Autodesk Inventor part; units mm, degrees
ref_plane "YZ Plane" through (0, 0, 0) normal (1, 0, 0) x (0, 1, 0)
ref_plane "XZ Plane" through (0, 0, 0) normal (0, 1, 0) x (-1, 0, 0)
ref_plane "XY Plane" through (0, 0, 0) normal (0, 0, 1) x (1, 0, 0)
ref_plane "Work Plane1" through (469.0633, -361.0645, -298.4444) normal (0, 1, 0) x (0, 0, 1)
sketch "Sketch2" plane through (469.0633, -361.0645, -298.4444) normal (0, 1, 0) x (0, 0, 1)
  circle A0 centre (0, 0) radius 3
  point P0 (298.4444, -469.0633)
  dimension "d6" = 6
extrude "Extrusion1" add sketch "Sketch2" along normal blind 251
sketch "Sketch5" plane through (469.0633, -110.0645, -298.4444) normal (0, 1, 0) x (1, 0, 0)
  circle A0 centre (0, 0) radius 3
  circle A1 centre (0, 0) radius 1.5
  point P0 (-469.0633, -298.4444)
  dimension "d26" = 3
extrude "Extrusion2" add sketch "Sketch5" along normal blind 4.7 contours A1
sketch "Sketch6" plane through (469.0633, -105.3645, -298.4444) normal (0, 1, 0) x (1, 0, 0)
  circle A0 centre (0, 0) radius 1.5
  circle A1 centre (0, 0) radius 2
  point P0 (-469.0633, -298.4444)
  dimension "d29" = 4
extrude "Extrusion3" add sketch "Sketch6" against normal blind 3.7
thread "Thread1"
chamfer "Chamfer2" distance 0.3 angle 45 1 edges at (467.0633, -105.3645, -298.4444)
sketch "Sketch7" plane through (469.0633, -361.0645, -298.4444) normal (0, -1, 0) x (1, 0, 0)
  circle A0 centre (0, 0) radius 3
  circle A1 centre (0, 0) radius 1.5
  point P0 (-469.0633, 298.4444)
  dimension "d37" = 3
extrude "Extrusion4" add sketch "Sketch7" along normal blind 4.7 contours A1
sketch "Sketch8" plane through (469.0633, -365.7645, -298.4444) normal (0, -1, 0) x (1, 0, 0)
  circle A0 centre (0, 0) radius 1.5
  circle A1 centre (0, 0) radius 2
  point P0 (-469.0633, 298.4444)
  dimension "d40" = 4
extrude "Extrusion5" add sketch "Sketch8" against normal blind 3.7
thread "Thread2"
chamfer "Chamfer3" distance 0.3 angle 45 1 edges at (467.0633, -365.7645, -298.4444)
properties material "Aluminum 6061"
Input: part model. Units: mm. Frame: model coordinates. A direction names the side the tool comes from. Coordinates: 2 decimals unless noted, no trailing zeros. Loops run counter-clockwise (first coordinate to the right, second up) from the corner with the lowest first, then second, coordinate; pieces in that order, holes last. Notation, with made-up numbers: (77, -18.75) - (112, -18.75) arc R19 ccw to (112, 17.25) - close; hole circle Ø5 at (78, 23). An arc over 180 degrees is marked (long way). Answer in a Markdown table with one row per item.
(1) Material intervals for L1, parallel to Y at x = 469.95, z = -299.8; L2, parallel to Y at x = 470.95, z = -297.95; L3, parallel to Z at x = 471.3, y = -279.5, sorted ascending. Write a range as from..to.
Model answer:
| item | result |
|---|---|
| L1 | y = -365.76..-362.06, -361.06..-110.06, -109.06..-105.36 |
| L2 | y = -365.51..-362.06, -361.06..-110.06, -109.06..-105.61 |
| L3 | z = -300.44..-296.45 |
(2) Set-up query: faces 1 (the face through (470.97, -107.34, -299.05)), 2 (the face through (468, -361.064, -300)), 3 (the face through (470.97, -363.79, -297.84)). Return all of +Z, -Z, +X, -X, +Y, -Y with unobstructed straight access to the full face (end or side cutting, diameter ignored); none if empty.
Model answer:
| item | result |
|---|---|
| face 1 | +Y |
| face 2 | none |
| face 3 | -Y |
(3) Pin query (flat end, axial travel): P1, Ø1, axis at x = 470.5, y = -311.5, coming from the +Z side; P2, Ø1, axis at x = 468, y = -165, coming from the +Z side. Return the tip coordinate at first contact, or that it passes through.
Model answer:
| item | result |
|---|---|
| P1 | stops at z = -295.59 |
| P2 | stops at z = -295.5 |
(4) Mould query, pull axis Y, two halves, no side actions, for faces 4 (the face through (470, -109.064, -300)), 5 (the face through (468, -110.064, -300)), 6 (the face through (466.09, -237.32, -298.83)). Classes: pulls with the +Y half, pulls with the -Y half, needs draft (parallel to the pull), parting line crosses it, or undercut.
Model answer:
| item | result |
|---|---|
| face 4 | undercut |
| face 5 | undercut |
| face 6 | needs draft |
(5) Cut plane A-A on y = -303. Output: boundary loops of the cut face in (x, z), plus the area to 3 significant figures.
Model answer:
| item | result |
|---|---|
| outline | circle Ø6 at (469.06, -298.44) |
| area | 28.3 mm² |
